Print and shaded views of the part. All mm, measured from the part's lowest x, y and z. Coordinates: 2 decimals unless noted, no trailing zeros. Order: outer loops, then holes, each group sorted by start corner. A loop starts at its lowest first (then second) coordinate and runs counter-clockwise, first axis right, second up. Notation, with made-up numbers: (-0.75, 23.5) -> (14.25, 23.5) arc R16 ccw to (14.25, 40.5) -> close; hole circle Ø11 at (-26.5, 36). An arc over 180 degrees is marked (long way). Return JSON: item names as keys, results as strings. Group by question number.
1) Cut at B-B (z = 0.6). Write the cut outline in (x, y) (3 decimals), and give its area (3 significant figures).
2) Cut at A-A (x = 66.5). Write the cut outline in (y, z), and give its area (3 significant figures).
3) Flat gauge pins, fed straight in: pin 1 (1 mm diameter, centred on y = 4.5, z = 1.5, fed in from -X); pin 2 (1.5 mm diameter, centred on x = 56, z = 2, fed in from +Y). Where does each tip first touch, or does it go through?
4) Probe line 1 (X direction, y = 9.5, z = 2.45); line 2 (X direction, y = 11, z = 0.7); line 3 (X direction, y = 8, z = 2.2). List the from-to ranges inside material, lowest first.
5) Cut at C-C (x = 23.5). Write the cut outline in (y, z).
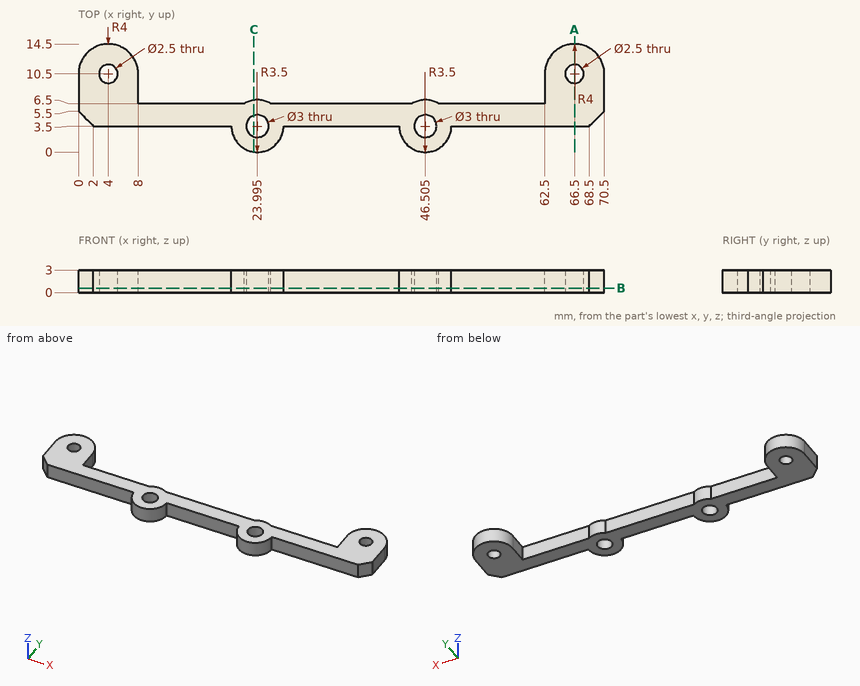
Answers below:
{
 "1": {"outline": "(0, 5.5) -> (2, 3.5) -> (20.495, 3.5) arc R3.5 ccw to (27.495, 3.5) -> (43.005, 3.5) arc R3.5 ccw to (50.005, 3.5) -> (68.5, 3.5) -> (70.5, 5.5) -> (70.5, 10.5) arc R4 ccw to (62.5, 10.5) -> (62.5, 6.5) -> (48.308, 6.5) arc R3.5 ccw to (44.702, 6.5) -> (25.798, 6.5) arc R3.5 ccw to (22.192, 6.5) -> (8, 6.5) -> (8, 10.5) arc R4 ccw to (0, 10.5) -> close; hole circle Ø2.5 at (4, 10.5); hole circle Ø3 at (23.995, 3.5); hole circle Ø3 at (46.505, 3.5); hole circle Ø2.5 at (66.5, 10.5)", "area": "339 mm^2"},
 "2": {"outline": "(3.5, 0) -> (9.25, 0) -> (9.25, 3) -> (3.5, 3) -> close; (11.75, 0) -> (14.5, 0) -> (14.5, 3) -> (11.75, 3) -> close", "area": "25.5 mm^2"},
 "3": {"pin 1": "stops at x = 0.5", "pin 2": "stops at y = 6.5"},
 "4": {"line 1": "x = 0 to 3.25, 4.75 to 8, 62.5 to 65.75, 67.25 to 70.5", "line 2": "x = 0.03 to 2.85, 5.15 to 7.97, 62.53 to 65.35, 67.65 to 70.47", "line 3": "x = 0 to 8, 62.5 to 70.5"},
 "5": {"outline": "(0.04, 0) -> (2.08, 0) -> (2.08, 3) -> (0.04, 3) -> close; (4.92, 0) -> (6.96, 0) -> (6.96, 3) -> (4.92, 3) -> close"}
}
